CAD build for the part. Positions are in the model's coordinates, mm. Face numbers are marked on the shaded views. Coordinates: 2 decimals unless noted, no trailing zeros. Order: outer loops, then holes, each group sorted by start corner. A loop starts at its lowest first (then second) coordinate and runs counter-clockwise, first axis right, second up. Notation, with made-up numbers: M -35,37.5 L -27,37.5 A18 ccw -27,44.5 Z; hole C 13.25,-38.5 d5. An arc over 180 degrees is marked long. One line per item, written item: value.
from build123d import *

# Parameters (mm, degrees)
SKETCH1_W          = 889
SKETCH1_H          = 31.75
EXTRUDE1_DEPTH     = 28.575
EXTRUDE2_REACH     = 891
SKETCH2_W          = 25.4
SKETCH2_H          = 25.4
HOLE1_D            = 6.35
HOLE1_DEPTH        = 3.175
LPATTERN1_COUNT    = 35
LPATTERN1_PITCH    = 25.4
HOLE2_D            = 9.652
HOLE2_DEPTH        = 3.175
LPATTERN2_COUNT    = 12
LPATTERN2_PITCH    = 25.4
HOLE3_D            = 9.652
HOLE3_DEPTH        = 3.175
HOLE4_D            = 9.652
HOLE4_DEPTH        = 3.175
LPATTERN3_COUNT    = 12
LPATTERN3_PITCH    = 25.4
HOLE5_D            = 3.175
HOLE5_DEPTH        = 3.175
HOLE6_D            = 6.35
HOLE6_DEPTH        = 3.175
LPATTERN4_COUNT    = 35
LPATTERN4_PITCH    = 25.4
FILLET1_R          = 3.175
FILLET2_R          = 3.175
FILLET3_R          = 6.35
FILLET4_R          = 6.35
SKETCH16_W         = 145.760071232
SKETCH16_H         = 71.504803879
CUT_EXTRUDE2_DEPTH = 75
SKETCH17_W         = 473.628565651
SKETCH17_H         = 66.908943447
CUT_EXTRUDE3_DEPTH = 186
SKETCH18_W         = 75.554715297
SKETCH18_H         = 79.695835758
CUT_EXTRUDE4_DEPTH = 29.575


with BuildPart() as part:
    # Sketch1 → Extrude1 (new body)
    with BuildSketch(Plane.XY.offset(3.175)):
        with Locations((428.480011997, 8.672957166)):
            Rectangle(SKETCH1_W, SKETCH1_H)
    extrude(amount=-EXTRUDE1_DEPTH)

    # Sketch2 → Extrude2 (cut, up to next)
    with BuildSketch(Plane.ZY.offset(16.019988003), mode=Mode.PRIVATE) as extrude2_sk1:
        with Locations((-12.7, 8.672957166)):
            Rectangle(SKETCH2_W, SKETCH2_H)
    extrude2_tool1 = extrude(extrude2_sk1.sketch, amount=-EXTRUDE2_REACH, mode=Mode.PRIVATE) & part.part
    add(extrude2_tool1.solids().sort_by_distance((-16.019988, 8.672957, -12.7))[0], mode=Mode.SUBTRACT)

    # Hole1
    with Locations(Plane(origin=(0, 24.547957166, 0), x_dir=(-1, 0, 0), z_dir=(0, 1, 0))):
        with Locations((3.319988003, -12.7)):
            hole1 = Hole(HOLE1_D / 2, depth=HOLE1_DEPTH)

    # LPattern1: Hole1 ×35
    with Locations(*[(i * LPATTERN1_PITCH, 0, 0) for i in range(1, LPATTERN1_COUNT)]):
        add(hole1, mode=Mode.SUBTRACT)

    # Hole2
    with Locations(Plane.XY.offset(3.175)):
        with Locations((66.530011997, 10.577957166)):
            hole2 = Hole(HOLE2_D / 2, depth=HOLE2_DEPTH)

    # LPattern2: Hole2 ×12, 8 skipped
    with Locations(*[(i * LPATTERN2_PITCH, 0, 0) for i in range(1, LPATTERN2_COUNT) if i not in (2, 3, 4, 5, 6, 7, 8, 9)]):
        add(hole2, mode=Mode.SUBTRACT)

    # Hole3
    with Locations(Plane.XY.offset(3.175)):
        with Locations((428.480011997, 6.767957166)):
            Hole(HOLE3_D / 2, depth=HOLE3_DEPTH)

    # Hole4
    with Locations(Plane.XY.offset(3.175)):
        with Locations((511.030011997, 10.577957166)):
            hole4 = Hole(HOLE4_D / 2, depth=HOLE4_DEPTH)

    # LPattern3: Hole4 ×12, 8 skipped
    with Locations(*[(i * LPATTERN3_PITCH, 0, 0) for i in range(1, LPATTERN3_COUNT) if i not in (2, 3, 4, 5, 6, 7, 8, 9)]):
        add(hole4, mode=Mode.SUBTRACT)

    # Hole5
    with Locations(Plane.XY.offset(3.175)):
        with Locations((669.780011997, 8.672957166)):
            Hole(HOLE5_D / 2, depth=HOLE5_DEPTH)

    # Hole6
    with Locations(Plane(origin=(0, -4.027042834, 0), x_dir=(-1, 0, 0), z_dir=(0, 1, 0))):
        with Locations((3.319988003, -12.7)):
            hole6 = Hole(HOLE6_D / 2, depth=HOLE6_DEPTH)

    # LPattern4: Hole6 ×35
    with Locations(*[(i * LPATTERN4_PITCH, 0, 0) for i in range(1, LPATTERN4_COUNT)]):
        add(hole6, mode=Mode.SUBTRACT)

    # Fillet1
    fillet1_edges = [part.edges().sort_by_distance(p)[0] for p in [
        (428.480011997, 21.372957166, 0),
    ]]
    fillet(fillet1_edges, radius=FILLET1_R)

    # Fillet2
    fillet2_edges = [part.edges().sort_by_distance(p)[0] for p in [
        (428.480011997, -4.027042834, 0),
    ]]
    fillet(fillet2_edges, radius=FILLET2_R)

    # Fillet3
    fillet3_edges = [part.edges().sort_by_distance(p)[0] for p in [
        (428.480011997, -7.202042834, 3.175),
    ]]
    fillet(fillet3_edges, radius=FILLET3_R)

    # Fillet4
    fillet4_edges = [part.edges().sort_by_distance(p)[0] for p in [
        (428.480011997, 24.547957166, 3.175),
    ]]
    fillet(fillet4_edges, radius=FILLET4_R)

    # Sketch16 → Cut-Extrude2 (cut)
    with BuildSketch(Plane(origin=(0, 24.547957166, 0), x_dir=(1, 0, 0), z_dir=(0, 1, 0))):
        with Locations((40.099976381, -10.352401939)):
            Rectangle(SKETCH16_W, SKETCH16_H)
    extrude(amount=-CUT_EXTRUDE2_DEPTH, mode=Mode.SUBTRACT)

    # Sketch17 → Cut-Extrude3 (cut)
    with BuildSketch(Plane(origin=(0, 24.547957166, 0), x_dir=(1, 0, 0), z_dir=(0, 1, 0))):
        with Locations((288.165729172, -8.054471723)):
            Rectangle(SKETCH17_W, SKETCH17_H)
    extrude(amount=-CUT_EXTRUDE3_DEPTH, mode=Mode.SUBTRACT)

    # Sketch18 → Cut-Extrude4 (cut, through all)
    with BuildSketch(Plane.XY.offset(3.175)):
        with Locations((546.702654349, 2.856578578)):
            Rectangle(SKETCH18_W, SKETCH18_H)
    extrude(amount=-CUT_EXTRUDE4_DEPTH, mode=Mode.SUBTRACT)


solid = part.part
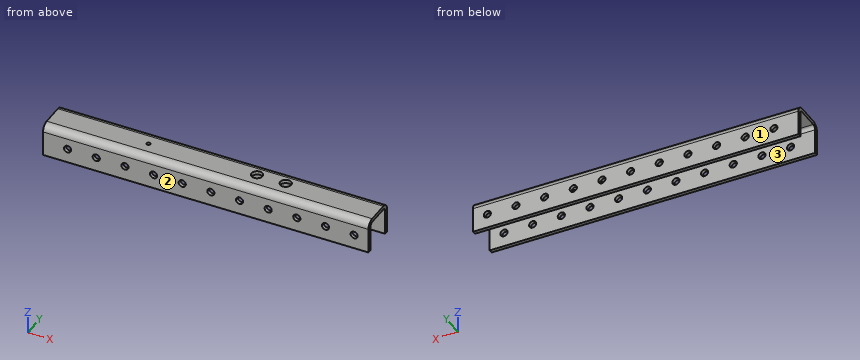
Q1. Slice it at B-B (x = 790). List the corners of the cut face in (y, z) (3 decimals).
Recorded:
outline: M -7.202,-25.4 L -4.027,-25.4 L -4.027,-3.175 A3.175 cw -0.852,0 L 5.771,0 L 5.771,3.175 L -0.852,3.175 A6.35 ccw -7.202,-3.175 Z; M 15.385,0 L 18.198,0 A3.175 cw 21.373,-3.175 L 21.373,-25.4 L 24.548,-25.4 L 24.548,-3.175 A6.35 ccw 18.198,3.175 L 15.385,3.175 Z
Q2. Mould opens along Y. For the marked faces 1, 2 and 3 say: released by +Y, released by -Y, zero draft, split by the parting line, or undercut.
Recorded:
face 1: released by +Y
face 2: released by -Y
face 3: undercut
Q3. Slice it at A-A (z = -6). List the corners of the cut face in (x, y), plus the area to 3 significant figures.
Recorded:
outline: M 584.48,-7.2 L 872.98,-7.2 L 872.98,-4.03 L 584.48,-4.03 Z; M 584.48,21.37 L 872.98,21.37 L 872.98,24.55 L 584.48,24.55 Z
area: 1,830 mm^2
Q4. Drill centre lines: line 1 along Y through (x, z) = (664.5, -18.75); line 2 along Z through (x, y) = (737.5, 6) (3 decimals); line 3 along Z through (x, y) = (801, 19). Where is each one in solid material? Low to high.
Recorded:
line 1: y = -7.2 to -4.03, 21.37 to 24.55
line 2: z = 0 to 3.175
line 3: z = -0.1 to 3.12
Q5. Pin check, flat tips, straight feed: pin 1 Ø1.5 at (x, z) = (713.5, -2) entering from +Y; pin 2 Ø15.5 at (x, y) = (765.03, 10.58) entering from -Z; pin 3 Ø2 at (x, y) = (703.5, -1.5) entering from -Z. Stop position of each tip, or through.
Recorded:
pin 1: stops at y = 24.53
pin 2: stops at z = 0
pin 3: stops at z = -0.46
